Work out the finished part from the listing and answer in its coordinate system (mm). Coordinates: 2 decimals unless noted, no trailing zeros. Order: outer loops, then holes, each group sorted by start corner. A loop starts at its lowest first (then second) coordinate and runs counter-clockwise, first axis right, second up. Notation, with made-up numbers: M 86.5,-11.5 L 138.5,-11.5 A17 ccw 138.5,-3.5 Z; hole C -7.75,22.5 d6. An arc over 180 degrees is marked long. Use a Markdown table: item, result.
from build123d import *

# Parameters (mm, degrees)
SKETCH_1_R          = 2.1
EXTRUDE_1_DEPTH     = 3
FILLET_2_R          = 3
SKETCH_3_R          = 1.6
SKETCH_3_R_2        = 2.1
CUT_EXTRUDE_2_DEPTH = 3


with BuildPart() as part:
    # 草图1 → 凸台-拉伸1 (new body)
    with BuildSketch(Plane.XY):
        Polygon((0, 0), (0, 31), (-28, 31), (-65.5, -33.951905284), (-183.57179677, -33.951905284), (-183.57179677, 36.048094716), (-198.57179677, 36.048094716), (-198.57179677, -45.951905284), (-58.57179677, -45.951905284), (-32.041451884, 0), align=None)
        with Locations((-6, 26)):
            Circle(SKETCH_1_R, mode=Mode.SUBTRACT)
        with Locations((-6, 6)):
            Circle(SKETCH_1_R, mode=Mode.SUBTRACT)
    extrude(amount=EXTRUDE_1_DEPTH)

    # 圆角2
    fillet_2_edges = [part.edges().sort_by_distance(p)[0] for p in [
        (-32.041451884, 0, 1.5),
        (-58.57179677, -45.951905284, 1.5),
        (-198.57179677, -45.951905284, 1.5),
        (-198.57179677, 36.048094716, 1.5),
        (-183.57179677, 36.048094716, 1.5),
        (-183.57179677, -33.951905284, 1.5),
        (-65.5, -33.951905284, 1.5),
        (-28, 31, 1.5),
        (0, 31, 1.5),
        (0, 0, 1.5),
    ]]
    fillet(fillet_2_edges, radius=FILLET_2_R)

    # 草图3 → 切除-拉伸2 (cut)
    with BuildSketch(Plane.XY.offset(3)):
        with Locations((-41.279056191, -4)):
            Circle(SKETCH_3_R)
        with Locations((-51.279056191, -21.320508076)):
            Circle(SKETCH_3_R)
        with Locations((-73.57179677, -39.951905284)):
            Circle(SKETCH_3_R)
        with Locations((-103.57179677, -39.951905284)):
            Circle(SKETCH_3_R)
        with Locations((-133.57179677, -39.951905284)):
            Circle(SKETCH_3_R)
        with Locations((-191.07179677, -19.951905284)):
            Circle(SKETCH_3_R_2)
        with Locations((-191.07179677, 5.048094716)):
            Circle(SKETCH_3_R_2)
        with Locations((-191.07179677, 30.048094716)):
            Circle(SKETCH_3_R_2)
        with Locations((-191.07179677, -39.951905284)):
            Circle(SKETCH_3_R_2)
        with Locations((-163.57179677, -39.951905284)):
            Circle(SKETCH_3_R)
    extrude(amount=-CUT_EXTRUDE_2_DEPTH, mode=Mode.SUBTRACT)


solid = part.part
(1) Straight lines are drawn through the part: L1, parallel to X at y = 25.5, z = 1.8; L2, parallel to X at y = -19, z = 1.1; L3, parallel to Y at x = -118.5, z = 1.05. For each, find the intervals that lie inside material, in ascending order.
Conclusion:
| item | result |
|---|---|
| L1 | -198.57 to -183.57, -31.18 to -8.04, -3.96 to 0 |
| L2 | -198.57 to -192.94, -189.2 to -183.57, -56.87 to -43.01 |
| L3 | -45.95 to -33.95 |
(2) A cutting plane is placed at D-D (y = -13.5). Determine the outline of the cut face in (x, z).
Conclusion:
| item | result |
|---|---|
| outline | M -198.57,0 L -183.57,0 L -183.57,3 L -198.57,3 Z; M -53.69,0 L -39.84,0 L -39.84,3 L -53.69,3 Z |
(3) A cutting plane is placed at A-A (x = -6). Determine the outline of the cut face in (y, z), then the cut area to 3 significant figures.
Conclusion:
| item | result |
|---|---|
| outline | M 0,0 L 3.9,0 L 3.9,3 L 0,3 Z; M 8.1,0 L 23.9,0 L 23.9,3 L 8.1,3 Z; M 28.1,0 L 31,0 L 31,3 L 28.1,3 Z |
| area | 67.8 mm2 |
(4) Determine the mould class of faces 1 (the flat face through (-45.48, -23.28, 1.48)), 2 (the flat face through (-46.5, -1.04, 1.48)), 3 (the flat face through (-107, -35, 3)) for opening direction X: pulls with the +X half, pulls with the -X half, needs draft (parallel to the pull), parting line crosses it, or undercut.
Conclusion:
| item | result |
|---|---|
| face 1 | pulls with the +X half |
| face 2 | undercut |
| face 3 | needs draft |
(5) A cutting plane is placed at C-C (z = 1.65). Give the number of separate pieces and of enclosed holes in the cut face, then the cut area to 3 significant figures.
Conclusion:
| item | result |
|---|---|
| separate pieces | 1 |
| enclosed holes | 12 |
| area | 4,250 mm2 |
(6) A cutting plane is placed at B-B (y = 26). Determine the outline of the cut face in (x, z).
Conclusion:
| item | result |
|---|---|
| outline | M -198.57,0 L -183.57,0 L -183.57,3 L -198.57,3 Z; M -30.89,0 L -8.1,0 L -8.1,3 L -30.89,3 Z; M -3.9,0 L 0,0 L 0,3 L -3.9,3 Z |
